```python
from build123d import *

# Parameters (mm, degrees)
SKETCH5_R           = 18.9865
BOSS_EXTRUDE3_DEPTH = 0.9906
SKETCH6_R           = 4.3434
CUT_EXTRUDE2_DEPTH  = 27.869232458
CUT_EXTRUDE3_DEPTH  = 27.869232458


with BuildPart() as part:
    # Sketch5 → Boss-Extrude3 (new body)
    with BuildSketch(Plane(origin=(0, 0, 0), x_dir=(1, 0, 0), z_dir=(0, 1, 0))):
        with Locations(Location((0, 0, 0), (0, 0, 270))):
            Circle(SKETCH5_R)
    extrude(amount=BOSS_EXTRUDE3_DEPTH)

    # Sketch6 → Cut-Extrude2 (cut, through all)
    with BuildSketch(Plane(origin=(0, 0.9906, 0), x_dir=(1, 0, 0), z_dir=(0, 1, 0))):
        with Locations(Location((0, 0, 0), (0, 0, 270))):
            Circle(SKETCH6_R)
    extrude(amount=-CUT_EXTRUDE2_DEPTH, mode=Mode.SUBTRACT)

    # Sketch7 → Cut-Extrude3 (cut, through all)
    with BuildSketch(Plane(origin=(0, 0.9906, 0), x_dir=(1, 0, 0), z_dir=(0, 1, 0))):
        with BuildLine():
            Line((-3.48206546, -18.664468982), (16.20193564, -9.898710207))
            ThreePointArc((16.20193564, -9.898710207), (7.723885426, -17.344416282), (-3.48206546, -18.664468982))
        make_face()
    extrude(amount=-CUT_EXTRUDE3_DEPTH, mode=Mode.SUBTRACT)


solid = part.part
```
Check sheet for the modelled part. Datum: model origin and axes. Units: mm. Coordinates: 2 decimals unless noted, no trailing zeros. Order: outer loops, then holes, each group sorted by start corner. A loop starts at its lowest first (then second) coordinate and runs counter-clockwise, first axis right, second up. Notation, with made-up numbers: M 45.5,4 L 88.5,4 A23 cw 88.5,16 Z; hole C 37.25,-6.75 d11. An arc over 180 degrees is marked long. One line per question, with ' | ' between items. Start each with the question number.
Item 1: Sectioned sample at A-A on x = 0. Record the cut outline in (y, z), and give its area (3 significant figures).
Item 2: Mould release check, pull along X, two halves, no side actions. Record for faces 1 (the flat face through (0, 0.991, -5)), 2 (the cylindrical face through (1.305, 0.502, 4.143)), 3 (the flat face through (6.222, 0.502, 14.343)): pulls with the +X half, pulls with the -X half, needs draft (parallel to the pull), parting line crosses it, or undercut.
Item 3: Sectioned sample at B-B on z = -3. Record the cut outline in (x, y).
Item 4: Sectioned sample at C-C on y = 0.8. Record the cut outline in (x, z), and give its area (3 significant figures).
Item 5: Material ranges on line 1 (X direction, y = 0.7, z = 0); line 2 (Z direction, x = 2, y = 0.75); line 3 (X direction, y = 0.7, z = 3.5), recorded low to high.
Item 6: Sectioned sample at D-D on z = 15.5. Record the cut outline in (x, y), and give its area (3 significant figures).
Answer below:
1) outline: M 0,-18.99 L 0.99,-18.99 L 0.99,-4.34 L 0,-4.34 Z; M 0,4.34 L 0.99,4.34 L 0.99,17.11 L 0,17.11 Z | area: 27.2 mm^2
2) face 1: needs draft | face 2: undercut | face 3: pulls with the +X half
3) outline: M -18.75,0 L -3.14,0 L -3.14,0.99 L -18.75,0.99 Z; M 3.14,0 L 18.75,0 L 18.75,0.99 L 3.14,0.99 Z
4) outline: M -3.48,18.66 A18.99 ccw long 16.2,9.9 Z; hole C 0,0 d8.69 | area: 1,020 mm^2
5) line 1: x = -18.99 to -4.34, 4.34 to 18.99 | line 2: z = -18.88 to -3.86, 3.86 to 16.22 | line 3: x = -18.66 to -2.57, 2.57 to 18.66
6) outline: M -10.97,0 L 3.62,0 L 3.62,0.99 L -10.97,0.99 Z | area: 14.5 mm^2
